CAD build for the part. Positions are in the model's coordinates, mm. Face numbers are marked on the shaded views. A direction names the side the tool comes from. Give positions to 0.01 mm unless a question says otherwise; leave off trailing zeros. Loops run counter-clockwise (first coordinate to the right, second up) from the corner with the lowest first, then second, coordinate; pieces in that order, holes last.
Item 1: Saw through at D-D on y = 28.5. Give the cut face in (x, z) (3 decimals), plus the area to 3 significant figures.
Item 2: Saw through at A-A on z = -4.5. Give the cut face in (x, y), plus the area to 3 significant figures.
Item 3: Drop flat-ended pins along their axis: P1, Ø10, axis at x = -10.5, z = -6, coming from the -Y side; P2, Ø4, axis at x = -12, y = 29, coming from the +Z side; P3, Ø6.5, axis at x = 1.5, y = 0.5, coming from the +Z side. Give the stop position or say it passes through.
Item 4: Which spindle directions (+Z, -Z, +X, -X, +Y, -Y) get a long thin tool onto all of the face, cutting with end or side? Do the marked faces 4, 5, 6, 7 and 8. Say none if no direction does.
Item 5: Mould opens along Y. For the marked faces 1, 2 and 3 say: released by +Y, released by -Y, zero draft, split by the parting line, or undercut.
Item 6: Saw through at C-C on x = 0. Give the cut face in (y, z), plus the area to 3 significant figures.
Item 7: Probe probe 1 along Y at (x, z) = (0, 3.85); probe 2 along X at (y, z) = (19.05, 4); probe 3 along Y at (x, z) = (1, 0.5). List the from-to ranges inside material, lowest first.
Item 8: Saw through at B-B on y = 19.05. Give the cut face in (x, z).
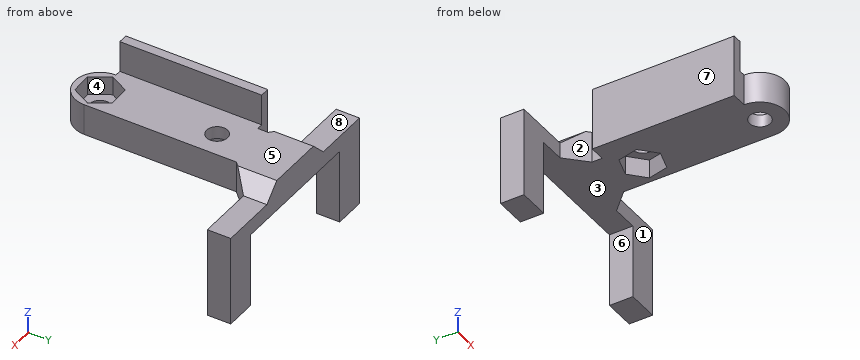
from build123d import *

# Parameters (mm, degrees)
SKETCH2_R           = 1.700000029
BOSS_EXTRUDE1_DEPTH = 5.08
SKETCH4_W           = 2.54
SKETCH4_H           = 23.100716355
BOSS_EXTRUDE3_DEPTH = 5.08
BOSS_EXTRUDE4_START = -5.08
SKETCH4_4_W         = 1.54
SKETCH4_4_H         = 23.100716355
BOSS_EXTRUDE4_DEPTH = 5.08
CUT_EXTRUDE1_START  = -3.048
SKETCH5_R           = 1.700000029
CUT_EXTRUDE1_DEPTH  = 3.048
CUT_EXTRUDE2_DEPTH  = 3.048
BOSS_EXTRUDE5_DEPTH = 3.81
CHAMFER4_SIZE       = 3.175
CHAMFER5_SIZE       = 3.175


with BuildPart() as part:
    # Sketch2 → Boss-Extrude1 (new body)
    with BuildSketch(Plane.XY):
        with BuildLine():
            Line((-4.064, 19.05), (-4.064, 0))
            ThreePointArc((-4.064, 0), (0, -4.064), (4.064, 0))
            Line((4.064, 0), (4.064, 19.05))
            Line((4.064, 19.05), (4.064, 31.75))
            Line((4.064, 31.75), (-4.064, 31.75))
            Line((-4.064, 31.75), (-4.064, 19.05))
        make_face()
        Circle(SKETCH2_R, mode=Mode.SUBTRACT)
        with Locations((0, 19.05)):
            Circle(SKETCH2_R, mode=Mode.SUBTRACT)
    extrude(amount=BOSS_EXTRUDE1_DEPTH)

    # Sketch4 → Boss-Extrude3 (add)
    with BuildSketch(Plane(origin=(0, 0, 0), x_dir=(-1, 0, 0), z_dir=(0, 0, -1))):
        with Locations((5.334, 11.550358178)):
            Rectangle(SKETCH4_W, SKETCH4_H)
    extrude(amount=-BOSS_EXTRUDE3_DEPTH)

    # Sketch4<4> → Boss-Extrude4 (add)
    with BuildSketch(Plane(origin=(0, 0, 0), x_dir=(-1, 0, 0), z_dir=(0, 0, -1)).offset(BOSS_EXTRUDE4_START)):
        with Locations((5.834, 11.550358178)):
            Rectangle(SKETCH4_4_W, SKETCH4_4_H)
    extrude(amount=-BOSS_EXTRUDE4_DEPTH)

    # Sketch5 → Cut-Extrude1 (cut)
    with BuildSketch(Plane.XY.offset(5.08).offset(CUT_EXTRUDE1_START)):
        Polygon((1.63025736, 3.061744972), (-1.836420245, 2.942716775), (-3.466677606, -0.119028197), (-1.63025736, -3.061744972), (1.836420245, -2.942716775), (3.466677606, 0.119028197), align=None)
        Circle(SKETCH5_R, mode=Mode.SUBTRACT)
    extrude(amount=CUT_EXTRUDE1_DEPTH, mode=Mode.SUBTRACT)

    # Sketch6 → Cut-Extrude2 (cut)
    with BuildSketch(Plane(origin=(0, 0, 0), x_dir=(-1, 0, 0), z_dir=(0, 0, -1))):
        Polygon((-3.253201396, 20.05995743), (-2.501249489, 16.737623663), (0.751951906, 15.727666232), (3.253201396, 18.04004257), (2.501249489, 21.362376337), (-0.751951906, 22.372333768), align=None)
    extrude(amount=-CUT_EXTRUDE2_DEPTH, mode=Mode.SUBTRACT)

    # Sketch9 → Boss-Extrude5 (add)
    with BuildSketch(Plane(origin=(0, 31.75, 0), x_dir=(1, 0, 0), z_dir=(0, 1, 0))):
        Polygon((-16.51, 12.065), (-16.51, -2.54), (16.51, -2.54), (16.51, 12.065), (11.43, 12.065), (11.43, 0), (-11.43, 0), (-11.43, 12.065), align=None)
    extrude(amount=-BOSS_EXTRUDE5_DEPTH)

    # Chamfer4
    # the kernel refuses this chamfer: 3.175 mm, written as the material it adds along each edge
    with BuildSketch(Plane(origin=(4.064, 27.94, 2.54), x_dir=(0.9996219169112966, 0, -0.02749587661058635), z_dir=(0, 1, 0))) as chamfer4_piece_1_section:
        Polygon((CHAMFER4_SIZE * 0.999621916911, -CHAMFER4_SIZE * 0.0274958766106), (-CHAMFER4_SIZE * 0.0274958766106, -CHAMFER4_SIZE * 0.999621916911), (0, 0), align=None)
    chamfer4_piece_1 = extrude(amount=3.81, mode=Mode.PRIVATE)
    chamfer4_piece_1 = split(chamfer4_piece_1, bisect_by=Plane(origin=(5.161655959, 29.845, 5.08), z_dir=(0, 0, -1)), keep=Keep.TOP, mode=Mode.PRIVATE)
    add(chamfer4_piece_1)
    with BuildSketch(Plane(origin=(-4.064, 31.75, 2.54), x_dir=(0.02749587661058607, 0, 0.9996219169112968), z_dir=(0, -1, 0))) as chamfer4_piece_2_section:
        Polygon((CHAMFER4_SIZE * 0.999621916911, CHAMFER4_SIZE * 0.0274958766106), (-CHAMFER4_SIZE * 0.0274958766106, CHAMFER4_SIZE * 0.999621916911), (0, 0), align=None)
    chamfer4_piece_2 = extrude(amount=3.81, mode=Mode.PRIVATE)
    chamfer4_piece_2 = split(chamfer4_piece_2, bisect_by=Plane(origin=(-5.161655959, 29.845, 5.08), z_dir=(0, 0, -1)), keep=Keep.TOP, mode=Mode.PRIVATE)
    add(chamfer4_piece_2)

    # Chamfer5
    chamfer5_edges = [part.edges().sort_by_distance(p)[0] for p in [
        (4.064, 27.94, 2.54),
        (-4.064, 27.94, 2.54),
    ]]
    chamfer(chamfer5_edges, length=CHAMFER5_SIZE)


solid = part.part
Results below:
1. outline: (-16.51, -12.065) - (-11.43, -12.065) - (-11.43, 0) - (11.43, 0) - (11.43, -12.065) - (16.51, -12.065) - (16.51, 2.54) - (7.239, 2.54) - (4.699, 5.08) - (-4.699, 5.08) - (-7.239, 2.54) - (-16.51, 2.54) - close
1. area: 237 mm2
2. outline: (-16.51, 27.94) - (-11.43, 27.94) - (-11.43, 31.75) - (-16.51, 31.75) - close; (11.43, 27.94) - (16.51, 27.94) - (16.51, 31.75) - (11.43, 31.75) - close
2. area: 38.7 mm2
3. P1: stops at y = 27.94
3. P2: stops at z = 2.54
3. P3: stops at z = 5.08
4. face 4: +Z
4. face 5: +Z, +X, +Y, -Y
4. face 6: -Z, +Y, -Y
4. face 7: +Z, -Z, -X, -Y
4. face 8: +Z, -X, +Y, -Y
5. face 1: released by -Y
5. face 2: undercut
5. face 3: zero draft
6. outline: (-4.06, 0) - (-1.7, 0) - (-1.7, 2.03) - (-3.01, 2.03) - (-3.01, 5.08) - (-4.06, 5.08) - close; (1.7, 0) - (15.96, 0) - (15.96, 3.05) - (17.35, 3.05) - (17.35, 5.08) - (3.01, 5.08) - (3.01, 2.03) - (1.7, 2.03) - close; (20.75, 3.05) - (22.14, 3.05) - (22.14, 0) - (31.75, 0) - (31.75, 5.08) - (20.75, 5.08) - close
6. area: 131 mm2
7. probe 1: y = -4.06 to -3.01, 3.01 to 17.35, 20.75 to 31.75
7. probe 2: x = -6.6 to -1.7, 1.7 to 4.06
7. probe 3: y = -3.94 to -1.37, 1.37 to 16.27, 22.14 to 31.75
8. outline: (-6.6, 0) - (-3.02, 0) - (-3.02, 3.05) - (-1.7, 3.05) - (-1.7, 5.08) - (-5.06, 5.08) - (-5.06, 10.16) - (-6.6, 10.16) - close; (1.7, 3.05) - (3.02, 3.05) - (3.02, 0) - (4.06, 0) - (4.06, 5.08) - (1.7, 5.08) - close
